Source: three-view drawing plus pictorial views. Frame: mm from the lowest corner of the part. A direction names the side the tool comes from. Round coordinates to 2 decimals unless told otherwise and drop trailing zeros. Loops run counter-clockwise (first coordinate to the right, second up) from the corner with the lowest first, then second, coordinate; pieces in that order, holes last. Notation, with made-up numbers: (77.25, 11.25) -> (85.25, 11.25) arc R19 cw to (85.25, 46.25) -> close; hole circle Ø5 at (6, -11.5). An arc over 180 degrees is marked (long way). Return JSON: item names as keys, results as strings. Group by question number.
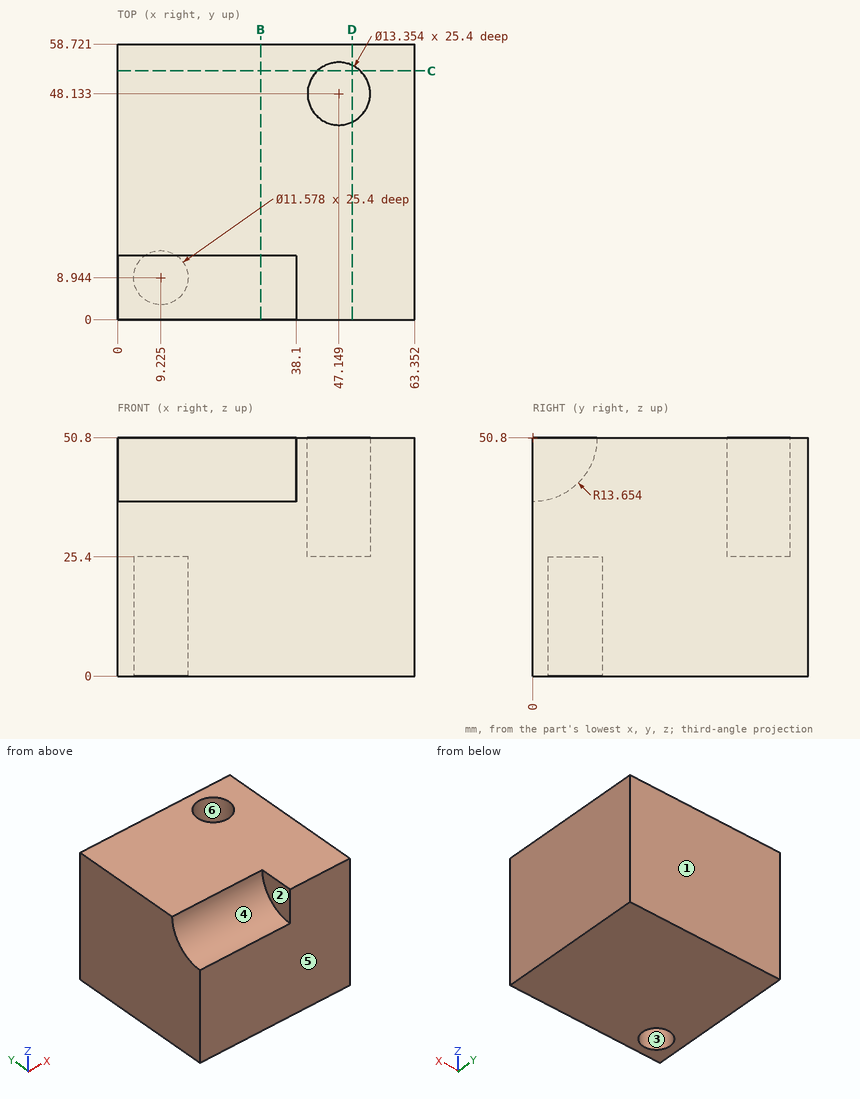
(1) Mould query, pull axis Y, two halves, no side actions, for the marked faces 1, 2 and 3. Classes: released by +Y, released by -Y, zero draft, split by the parting line, or undercut.
(2) Cut plane C-C (y = 53). Return loops of the section in (x, z), and give its area (3 significant figures).
(3) Ray query, line 1 (X direction, y = 49, z = 29); line 2 (Z direction, x = 48.5, y = 46); line 3 (Y direction, x = 11.5, z = 5.5). Return the intervals inside material, ascending.
(4) Pin query (flat end, axial travel): pin 1 (10.5 mm diameter, centred on x = 9.23, y = 8.94, fed in from -Z). Return the tip coordinate at first contact, or that it passes through.
(5) Cut plane B-B (x = 30.5). Return loops of the section in (y, z).
(6) Set-up query: the marked faces 4, 5 and 6. Return all of +Z, -Z, +X, -X, +Y, -Y with unobstructed straight access to the full face (end or side cutting, diameter ignored); none if empty.
(7) Cut plane D-D (x = 50). Return loops of the section in (y, z) (1 decimal), and give its area (3 significant figures).
Answers follow:
{
 "1": {"face 1": "released by +Y", "face 2": "zero draft", "face 3": "undercut"},
 "2": {"outline": "(0, 0) -> (63.35, 0) -> (63.35, 50.8) -> (51.72, 50.8) -> (51.72, 25.4) -> (42.58, 25.4) -> (42.58, 50.8) -> (0, 50.8) -> close", "area": "2,990 mm^2"},
 "3": {"line 1": "0 to 40.53, 53.77 to 63.35", "line 2": "0 to 25.4", "line 3": "0 to 3.62, 14.27 to 58.72"},
 "4": {"pin 1": "z = 25.4"},
 "5": {"outline": "(0, 0) -> (58.72, 0) -> (58.72, 50.8) -> (13.65, 50.8) arc R13.65 cw to (0, 37.15) -> close"},
 "6": {"face 4": "+Z, -X, -Y", "face 5": "+Z, -Z, +X, -X, -Y", "face 6": "+Z"},
 "7": {"outline": "(0, 0) -> (58.7, 0) -> (58.7, 50.8) -> (54.2, 50.8) -> (54.2, 25.4) -> (42.1, 25.4) -> (42.1, 50.8) -> (0, 50.8) -> close", "area": "2,680 mm^2"}
}
